Geometry check sheet. Reference: the model listing, model coordinates, mm. Round coordinates to 2 decimals unless told otherwise and drop trailing zeros. Return JSON: item names as keys, results as strings.
```python
from build123d import *

# Parameters (mm, degrees)
SKETCH1_W           = 355.6
SKETCH1_H           = 127
SKETCH1_R           = 9.525
SKETCH1_R_2         = 2.5527
BOSS_EXTRUDE1_DEPTH = 5.08
SKETCH2_W           = 355.6
SKETCH2_H           = 1016
BOSS_EXTRUDE2_DEPTH = 5.08
SKETCH4_R           = 1.5875
CUT_EXTRUDE1_DEPTH  = 6.08


with BuildPart() as part:
    # Sketch1 → Boss-Extrude1 (new body)
    with BuildSketch(Plane(origin=(0, 0, 0), x_dir=(1, 0, 0), z_dir=(0, 1, 0))):
        Rectangle(SKETCH1_W, SKETCH1_H)
        Circle(SKETCH1_R, mode=Mode.SUBTRACT)
        with Locations((12.5, 21.650635095)):
            Circle(SKETCH1_R_2, mode=Mode.SUBTRACT)
        with Locations((12.5, -21.650635095)):
            Circle(SKETCH1_R_2, mode=Mode.SUBTRACT)
        with Locations((-25, 0)):
            Circle(SKETCH1_R_2, mode=Mode.SUBTRACT)
    extrude(amount=BOSS_EXTRUDE1_DEPTH)

    # Sketch2 → Boss-Extrude2 (add)
    with BuildSketch(Plane(origin=(0, 5.08, 0), x_dir=(1, 0, 0), z_dir=(0, 1, 0))):
        with Locations((0, 571.5)):
            Rectangle(SKETCH2_W, SKETCH2_H)
    extrude(amount=-BOSS_EXTRUDE2_DEPTH)

    # Sketch4 → Cut-Extrude1 (cut, through all)
    with BuildSketch(Plane(origin=(0, 5.08, 0), x_dir=(1, 0, 0), z_dir=(0, 1, 0))):
        with Locations((11.1125, 1039.8125)):
            Circle(SKETCH4_R)
        with Locations((-11.1125, 1039.8125)):
            Circle(SKETCH4_R)
        with Locations((0, 1016)):
            Circle(SKETCH4_R)
    extrude(amount=-CUT_EXTRUDE1_DEPTH, mode=Mode.SUBTRACT)


solid = part.part
```
(1) Material ranges on line 1 along Z through (x, y) = (0, 1.65) (1 decimal); line 2 along Z through (x, y) = (12.5, 2.4), recorded low to high. Write a range as [from, to].
Response values:
{"line 1": "z = [-1079.5, -1017.6], [-1014.4, -9.5], [9.5, 63.5]", "line 2": "z = [-1079.5, -1040.58], [-1039.04, -24.2], [-19.1, 19.1], [24.2, 63.5]"}
(2) Gauge pin test, flat ends, axial feed: pin 1 (8 mm diameter, centred on x = 12.5, z = -21.65, fed in from +Y); pin 2 (17 mm diameter, centred on x = 0, z = 0, fed in from -Y). Record the tip position at first contact, or that the pin passes through.
Response values:
{"pin 1": "stops at y = 5.08", "pin 2": "passes through"}
(3) Release check for a two-part mould opening along X. For faces 1 (the face through (-2, 5.08, -516)), 2 (the face through (-7.559, 2.504, 5.796)) record: pulls with the +X half, pulls with the -X half, needs draft (parallel to the pull), parting line crosses it, or undercut.
Response values:
{"face 1": "needs draft", "face 2": "undercut"}
